Source: CAD feature listing. Evaluate the final solid. Frame: model axes, mm. Give positions to 0.01 mm unless a question says otherwise; leave off trailing zeros. Order: outer loops, then holes, each group sorted by start corner. A loop starts at its lowest first (then second) coordinate and runs counter-clockwise, first axis right, second up.
Autodesk Fusion 360 part; units mm, degrees
sketch "Sketch1" plane through (0, 0, 0) normal (1, 0, 0) x (0, 1, 0)
  line L0 (0, 0) -> (2.3094, 4)
  line L1 (2.3094, 4) -> (11.8094, 4)
  line L2 (11.8094, 4) -> (14.1188, 0)
  line L3 (14.1188, 0) -> (0, 0)
  dimension "d1" = 4
  dimension "d2" = 9.5
  dimension "d3" = 60
extrude "Extrude1" add sketch "Sketch1" along normal blind 12.5
chamfer "Chamfer1" distance 1 angle 45 1 edges at (12.5, 7.0594, 4)
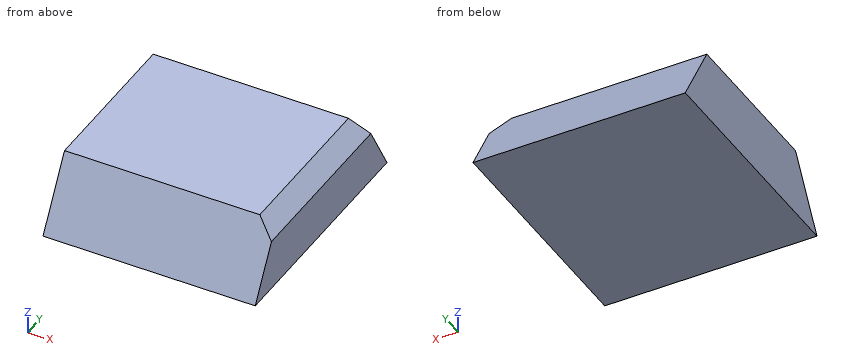
1) Section query A-A, the plane y = 12. Return the cut outline in (x, z).
Report:
outline: (0, 0) - (12.5, 0) - (12.5, 3) - (11.83, 3.67) - (0, 3.67) - close
2) Material intervals for L1, parallel to Z at x = 5.75, y = 1; L2, parallel to Y at x = 11.5, z = 3.2; L3, parallel to Z at x = 12, y = 11.5, sorted ascending.
Report:
L1: z = 0 to 1.73
L2: y = 1.85 to 12.27
L3: z = 0 to 3.5
3) Pin query (flat end, axial travel): pin 1 (2 mm diameter, centred on y = 1.5, z = 1, fed in from -X). Return the tip coordinate at first contact, or that it passes through.
Report:
pin 1: stops at x = 0
4) Section query C-C, the plane z = 2.7. Return the cut outline in (x, y).
Report:
outline: (0, 1.56) - (12.5, 1.56) - (12.5, 12.56) - (0, 12.56) - close
5) Section query B-B, the plane x = 5.5. Return the cut outline in (y, z).
Report:
outline: (0, 0) - (14.12, 0) - (11.81, 4) - (2.31, 4) - close
